Geometry check sheet. Reference: the model listing, model coordinates, mm. A direction names the side the tool comes from. Coordinates: 2 decimals unless noted, no trailing zeros. Answer in a Markdown table with one row per item. Add a question column.
1. Set-up check for faces 1 (the cylindrical face through (-7, 0, 23)), 2 (the cylindrical face through (1.617, -0.67, 30.43)), 3 (the cylindrical face through (7, 0, 23)), 4 (the flat face through (-8, 0, 5)), 5 (the cylindrical face through (-0.16, 11.65, 8.24)): record each of +Z, -Z, +X, -X, +Y, -Y from which the full face is reachable in a straight line by a thin tool's end or side.
2. Mould release check, pull along X, two halves, no side actions. Record for faces 6 (the flat face through (8, -2, 3)), 7 (the flat face through (5.5, 1, 25)), 8 (the cylindrical face through (-3.77, -0.27, 24.78)): pulls with the +X half, pulls with the -X half, needs draft (parallel to the pull), parting line crosses it, or undercut.
3. Depth check by flat-ended pin: P1, Ø1.8, axis at y = 0.5, z = 25, coming from the -X side; P2, Ø3, axis at x = 3.5, z = 10, coming from the -Y side; P3, Ø9, axis at x = 7.6, y = 0, coming from the -Z side. Enter the tip coordinate at first touch or a pass-through.
4. Scan lines: L1, parallel to X at y = 0, z = 4.5; L2, parallel to X at y = 0, z = 0.8; L3, parallel to Z at x = -4.65, y = 0. Record each from-to range of solid material in increasing order. Write a range as from..to.
```python
from build123d import *

# Parameters (mm, degrees)
F3_R          = 4
F4_DEPTH      = 3
F5_R          = 1.25
F6_DEPTH      = 2
F7_R          = 1.25
F8_DEPTH      = 2
F10_DEPTH     = 12.5
F11_T4_ANGLE  = 62.5690664244
F11_S5_R      = 10.55
F11_T6_DEPTH  = 7
F11_T10_ANGLE = 125.1442226545
F11_S11_R     = 10.55
F11_T12_DEPTH = 10
F11_T16_ANGLE = 62.5690664244
F11_S17_R     = 10.55
F11_T18_DEPTH = 7
F12_R         = 1.75
F13_DEPTH     = 3.5
F14_SIZE      = 0.6
F15_R         = 1.25
F16_DEPTH     = 3.3534363587
F19_R         = 1.25
F20_DEPTH     = 5
F21_R         = 3
F22_DEPTH     = 4.5
F23_R         = 1.25
F24_DEPTH     = 8
F25_R         = 3
F26_DEPTH     = 4.5


# Not quite as in the source:
# - a fillet or chamfer that OpenCascade refuses, or shapes differently, is made with other operations: its cross-section is extruded or revolved along the edge and cut away or added


with BuildPart() as f2:
    # F1 (on Front) → F2 (revolve)
    with BuildSketch(Plane.XZ):
        with BuildLine():
            Line((0, 29), (-7, 29))
            add(Edge.make_bspline(
                [(0, 0), (-5.317841365, 0), (-8.4305850004, 0.3570766518), (-14.8822587004, 4.4570633142), (-13.316672088, 15.36842657), (-7, 29)],
                knots=[0, 0, 0, 0, 0.2945682266, 0.5047389267, 1, 1, 1, 1], degree=3))
            Line((0, 0), (0, 29))
        make_face()
    revolve(axis=Axis((0, 0, 7.1166679263), (0, 0, -1)))

    # F3 (on Top) → F4 (cut)
    with BuildSketch(Plane.XY):
        with Locations((-7.6, 0)):
            Circle(F3_R)
        with Locations((7.6, 0)):
            Circle(F3_R)
    extrude(amount=F4_DEPTH, mode=Mode.SUBTRACT)

    # F5 (on face) → F6 (cut)
    with BuildSketch(Plane(origin=(0, 0, 3), x_dir=(1, 0, 0), z_dir=(0, 0, -1))):
        with Locations((7.6, 0)):
            Circle(F5_R)
    extrude(amount=-F6_DEPTH, mode=Mode.SUBTRACT)

    # F7 (on face) → F8 (cut)
    with BuildSketch(Plane(origin=(0, 0, 3), x_dir=(1, 0, 0), z_dir=(0, 0, -1))):
        with Locations((-7.6, 0)):
            Circle(F7_R)
    extrude(amount=-F8_DEPTH, mode=Mode.SUBTRACT)

    # F9 (on Right) → F10 (cut, symmetric)
    with BuildSketch(Plane.YZ):
        with BuildLine():
            Line((-10.1144698329, 31.8), (-10.1144698329, 21.8))
            ThreePointArc((-10.1144698329, 21.8), (0, 29.35), (10.1144698329, 21.8))
            Line((10.1144698329, 21.8), (10.1144698329, 31.8))
            Line((10.1144698329, 31.8), (-10.1144698329, 31.8))
        make_face()
    extrude(amount=F10_DEPTH, both=True, mode=Mode.SUBTRACT)

    # F11: fillet of radius 3 on 3 edges, made by hand


with BuildPart() as f11_tool2:
    # F11_s3 → F11_t4 (revolve)
    with BuildSketch(Plane.XZ):
        with BuildLine():
            ThreePointArc((-5.0697196206, 29), (-6.7017587776, 28.5172302616), (-7.8085318567, 27.2242987933))
            Line((-7.8085318567, 27.2242987933), (-7.8633081014, 27.2487847692))
            ThreePointArc((-7.8633081014, 27.2487847692), (-7.4618780859, 28.1383864481), (-7.0544392435, 29.0252263506))
            Line((-7.0544392435, 29.0252263506), (-7, 29.06))
            Line((-7, 29.06), (-5.0697196206, 29.06))
            Line((-5.0697196206, 29.06), (-5.0697196206, 29))
        make_face()
    revolve(axis=Axis((0, 0, 29), (0, 0, -1)), revolution_arc=F11_T4_ANGLE)

    # F11_s5 → F11_t6 (intersect, symmetric)
    with BuildSketch(Plane.YZ.offset(-5.5)):
        with Locations((0, 18.8)):
            Circle(F11_S5_R)
    extrude(amount=F11_T6_DEPTH, both=True, mode=Mode.INTERSECT)


with BuildPart() as f2_1:
    add(f2.part)

    # F11_t1: cut F11_tool2
    add(f11_tool2.part, mode=Mode.SUBTRACT)


with BuildPart() as f11_tool8:
    # F11_s9 → F11_t10 (revolve)
    with BuildSketch(Plane(origin=(0, 0, 0), x_dir=(0, 0, 1), z_dir=(-0.8875912781, 0.4606318736, 0))):
        with BuildLine():
            ThreePointArc((29, 5.0697196206), (28.5172302616, 6.7017587776), (27.2242987933, 7.8085318567))
            Line((27.2242987933, 7.8085318567), (27.2487847692, 7.8633081014))
            ThreePointArc((27.2487847692, 7.8633081014), (28.1383864481, 7.4618780859), (29.0252263506, 7.0544392435))
            Line((29.0252263506, 7.0544392435), (29.06, 7))
            Line((29.06, 7), (29.06, 5.0697196206))
            Line((29.06, 5.0697196206), (29, 5.0697196206))
        make_face()
    revolve(axis=Axis((0, 0, 29), (0, 0, -1)), revolution_arc=F11_T10_ANGLE)

    # F11_s11 → F11_t12 (intersect, symmetric)
    with BuildSketch(Plane.YZ.offset(5.3)):
        with Locations((0, 18.8)):
            Circle(F11_S11_R)
    extrude(amount=F11_T12_DEPTH, both=True, mode=Mode.INTERSECT)


with BuildPart() as f2_2:
    add(f2_1.part)

    # F11_t7: cut F11_tool8
    add(f11_tool8.part, mode=Mode.SUBTRACT)


with BuildPart() as f11_tool14:
    # F11_s15 → F11_t16 (revolve)
    with BuildSketch(Plane(origin=(0, 0, 0), x_dir=(0, 0, 1), z_dir=(0.8875667972, -0.4606790428, 0))):
        with BuildLine():
            ThreePointArc((29, 5.0697196206), (28.5172302616, 6.7017587776), (27.2242987933, 7.8085318567))
            Line((27.2242987933, 7.8085318567), (27.2487847692, 7.8633081014))
            ThreePointArc((27.2487847692, 7.8633081014), (28.1383864481, 7.4618780859), (29.0252263506, 7.0544392435))
            Line((29.0252263506, 7.0544392435), (29.06, 7))
            Line((29.06, 7), (29.06, 5.0697196206))
            Line((29.06, 5.0697196206), (29, 5.0697196206))
        make_face()
    revolve(axis=Axis((0, 0, 29), (0, 0, -1)), revolution_arc=F11_T16_ANGLE)

    # F11_s17 → F11_t18 (intersect, symmetric)
    with BuildSketch(Plane.YZ.offset(-5.5)):
        with Locations((0, 18.8)):
            Circle(F11_S17_R)
    extrude(amount=F11_T18_DEPTH, both=True, mode=Mode.INTERSECT)


with BuildPart() as f2_3:
    add(f2_2.part)

    # F11_t13: cut F11_tool14
    add(f11_tool14.part, mode=Mode.SUBTRACT)

    # F12 (on face) → F13 (join)
    with BuildSketch(Plane.XY.offset(29)):
        Circle(F12_R)
    extrude(amount=F13_DEPTH)

    # F14
    f14_edges = [f2_3.edges().sort_by_distance(p)[0] for p in [
        (-1.75, 0, 32.5),
    ]]
    chamfer(f14_edges, length=F14_SIZE)

    # F15 (on offset) → F16 (cut, through all)
    with BuildSketch(Plane.XZ.offset(-10)):
        with Locations((0, 7)):
            Circle(F15_R)
    extrude(amount=-F16_DEPTH, mode=Mode.SUBTRACT)

    # F19 (on offset) → F20 (cut)
    with BuildSketch(Plane.YZ.offset(10)):
        with Locations((0, 26)):
            Circle(F19_R)
    extrude(amount=-F20_DEPTH, mode=Mode.SUBTRACT)

    # F21 (on offset) → F22 (cut)
    with BuildSketch(Plane.YZ.offset(10)):
        with Locations((0, 26)):
            Circle(F21_R)
    extrude(amount=-F22_DEPTH, mode=Mode.SUBTRACT)

    # F23 (on offset) → F24 (cut)
    with BuildSketch(Plane.YZ.offset(-10)):
        with Locations((0, 26)):
            Circle(F23_R)
    extrude(amount=F24_DEPTH, mode=Mode.SUBTRACT)

    # F25 (on offset) → F26 (cut)
    with BuildSketch(Plane.YZ.offset(-10)):
        with Locations((0, 26)):
            Circle(F25_R)
    extrude(amount=F26_DEPTH, mode=Mode.SUBTRACT)


solid = f2_3.part
```
Results found:
| question | item | result |
|---|---|---|
| 1 | face 1 | -X |
| 1 | face 2 | +Z |
| 1 | face 3 | +X |
| 1 | face 4 | -Z |
| 1 | face 5 | +Y |
| 2 | face 6 | undercut |
| 2 | face 7 | pulls with the +X half |
| 2 | face 8 | needs draft |
| 3 | P1 | stops at x = -5.5 |
| 3 | P2 | stops at y = -13.14 |
| 3 | P3 | stops at z = 0.04 |
| 4 | L1 | x = -12.73..-8.85, -6.35..6.35, 8.85..12.73 |
| 4 | L2 | x = -3.6..3.6 |
| 4 | L3 | z = 3..24.75, 27.25..29 |
